Geometry: final body of the model. Coordinates: model frame, mm. Face numbers are marked on the shaded views. A direction names the side the tool comes from. Round coordinates to 2 decimals unless told otherwise and drop trailing zeros. Write each loop counter-clockwise with the first axis right and the second up, starting at its lowest first coordinate (ties: lowest second). Pieces come first, ordered by that corner, then holes. Notation, with made-up numbers: M 10.25,-19 L 40.25,-19 A14 cw 40.25,-6 Z; hole C -6.75,34 d4. An arc over 180 degrees is marked long. Put each result on its own line as item: value. Start each with the question number.
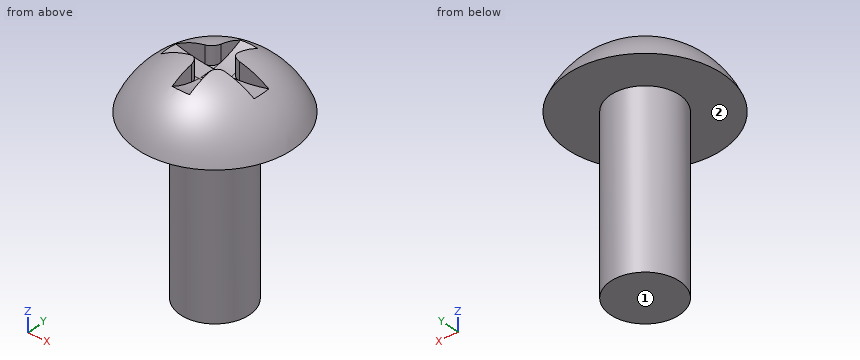
```python
from build123d import *

# Parameters (mm, degrees)
F0_R         = 2
F1_DEPTH     = 10
F5_DEPTH     = 0.5
F7_DEPTH     = 0.5
F8_T4_DEPTH  = 3.6233825309
F8_S5_R      = 10
F8_T6_DEPTH  = 3
F8_S7_R      = 5
F8_T8_DEPTH  = 3
F8_T12_DEPTH = 3.6233825309
F8_S13_R     = 10
F8_T14_DEPTH = 3
F8_S15_R     = 5
F8_T16_DEPTH = 3
F8_T20_DEPTH = 3.6233825309
F8_S21_R     = 10
F8_T22_DEPTH = 3
F8_S23_R     = 5
F8_T24_DEPTH = 3
F8_T28_DEPTH = 3.6233825309
F8_S29_R     = 10
F8_T30_DEPTH = 3
F8_S31_R     = 5
F8_T32_DEPTH = 3


# Not quite as in the source:
# - a fillet or chamfer that OpenCascade refuses, or shapes differently, is made with other operations: its cross-section is extruded or revolved along the edge and cut away or added


with BuildPart() as f1:
    # F0 (on Top) → F1 (new body)
    with BuildSketch(Plane.XY):
        Circle(F0_R)
    extrude(amount=F1_DEPTH)

    # F2 (on Front) → F3 (revolve)
    with BuildSketch(Plane.XZ):
        with BuildLine():
            Line((0, 10), (4.5, 10))
            ThreePointArc((4.5, 10), (2.7041634566, 12.1812451849), (0, 13))
            Line((0, 13), (0, 10))
        make_face()
    revolve(axis=Axis((0, 0, 12.25), (0, 0, -1)))

    # F4 (on Front) → F5 (cut, symmetric)
    with BuildSketch(Plane.XZ):
        with BuildLine():
            ThreePointArc((-2.7226391671, 12.177773856), (0, 11.8), (2.7226391671, 12.177773856))
            ThreePointArc((2.7226391671, 12.177773856), (0, 13), (-2.7226391671, 12.177773856))
        make_face()
    extrude(amount=F5_DEPTH, both=True, mode=Mode.SUBTRACT)

    # F6 (on Right) → F7 (cut, symmetric)
    with BuildSketch(Plane.YZ):
        with BuildLine():
            ThreePointArc((-2.3644931313, 12.3944157899), (0, 11.8), (2.3644931313, 12.3944157899))
            ThreePointArc((2.3644931313, 12.3944157899), (0, 13), (-2.3644931313, 12.3944157899))
        make_face()
    extrude(amount=F7_DEPTH, both=True, mode=Mode.SUBTRACT)

    # F8: fillet of radius 0.5 on 4 edges, made by hand


with BuildPart() as f8_tool2:
    # F8_s3 → F8_t4 (new body)
    with BuildSketch(Plane.XY.offset(10.5750628145)):
        with BuildLine():
            ThreePointArc((1, -0.5), (0.6464466094, -0.6464466094), (0.5, -1))
            Line((0.5, -1), (0.5, -0.5))
            Line((0.5, -0.5), (1, -0.5))
        make_face()
    extrude(amount=F8_T4_DEPTH)

    # F8_s5 → F8_t6 (intersect, symmetric)
    with BuildSketch(Plane.XZ.offset(0.8)):
        with Locations((0, 21.8)):
            Circle(F8_S5_R)
    extrude(amount=F8_T6_DEPTH, both=True, mode=Mode.INTERSECT)

    # F8_s7 → F8_t8 (intersect, symmetric)
    with BuildSketch(Plane.YZ.offset(0.8)):
        with Locations((0, 16.8)):
            Circle(F8_S7_R)
    extrude(amount=F8_T8_DEPTH, both=True, mode=Mode.INTERSECT)


with BuildPart() as f1_1:
    add(f1.part)

    # F8_t1: cut F8_tool2
    add(f8_tool2.part, mode=Mode.SUBTRACT)


with BuildPart() as f8_tool10:
    # F8_s11 → F8_t12 (new body)
    with BuildSketch(Plane.XY.offset(10.5750628145)):
        with BuildLine():
            ThreePointArc((-1, -0.5), (-0.6464466094, -0.6464466094), (-0.5, -1))
            Line((-0.5, -1), (-0.5, -0.5))
            Line((-0.5, -0.5), (-1, -0.5))
        make_face()
    extrude(amount=F8_T12_DEPTH)

    # F8_s13 → F8_t14 (intersect, symmetric)
    with BuildSketch(Plane.XZ.offset(0.8)):
        with Locations((0, 21.8)):
            Circle(F8_S13_R)
    extrude(amount=F8_T14_DEPTH, both=True, mode=Mode.INTERSECT)

    # F8_s15 → F8_t16 (intersect, symmetric)
    with BuildSketch(Plane.YZ.offset(-0.8)):
        with Locations((0, 16.8)):
            Circle(F8_S15_R)
    extrude(amount=F8_T16_DEPTH, both=True, mode=Mode.INTERSECT)


with BuildPart() as f1_2:
    add(f1_1.part)

    # F8_t9: cut F8_tool10
    add(f8_tool10.part, mode=Mode.SUBTRACT)


with BuildPart() as f8_tool18:
    # F8_s19 → F8_t20 (new body)
    with BuildSketch(Plane.XY.offset(10.5750628145)):
        with BuildLine():
            ThreePointArc((-1, 0.5), (-0.6464466094, 0.6464466094), (-0.5, 1))
            Line((-0.5, 1), (-0.5, 0.5))
            Line((-0.5, 0.5), (-1, 0.5))
        make_face()
    extrude(amount=F8_T20_DEPTH)

    # F8_s21 → F8_t22 (intersect, symmetric)
    with BuildSketch(Plane.XZ.offset(-0.7)):
        with Locations((0, 21.8)):
            Circle(F8_S21_R)
    extrude(amount=F8_T22_DEPTH, both=True, mode=Mode.INTERSECT)

    # F8_s23 → F8_t24 (intersect, symmetric)
    with BuildSketch(Plane.YZ.offset(-0.8)):
        with Locations((0, 16.8)):
            Circle(F8_S23_R)
    extrude(amount=F8_T24_DEPTH, both=True, mode=Mode.INTERSECT)


with BuildPart() as f1_3:
    add(f1_2.part)

    # F8_t17: cut F8_tool18
    add(f8_tool18.part, mode=Mode.SUBTRACT)


with BuildPart() as f8_tool26:
    # F8_s27 → F8_t28 (new body)
    with BuildSketch(Plane.XY.offset(10.5750628145)):
        with BuildLine():
            ThreePointArc((1, 0.5), (0.6464466094, 0.6464466094), (0.5, 1))
            Line((0.5, 1), (0.5, 0.5))
            Line((0.5, 0.5), (1, 0.5))
        make_face()
    extrude(amount=F8_T28_DEPTH)

    # F8_s29 → F8_t30 (intersect, symmetric)
    with BuildSketch(Plane.XZ.offset(-0.7)):
        with Locations((0, 21.8)):
            Circle(F8_S29_R)
    extrude(amount=F8_T30_DEPTH, both=True, mode=Mode.INTERSECT)

    # F8_s31 → F8_t32 (intersect, symmetric)
    with BuildSketch(Plane.YZ.offset(0.8)):
        with Locations((0, 16.8)):
            Circle(F8_S31_R)
    extrude(amount=F8_T32_DEPTH, both=True, mode=Mode.INTERSECT)


with BuildPart() as f1_4:
    add(f1_3.part)

    # F8_t25: cut F8_tool26
    add(f8_tool26.part, mode=Mode.SUBTRACT)


solid = f1_4.part
```
1) Section A-A, the plane y = -0.75. Output: boundary loops of the cut face in (x, z) (3 decimals).
2) Section D-D, the plane y = -1.75. Output: boundary loops of the cut face in (x, z) (3 decimals).
3) First-contact query: pin 1 (0.5 mm diameter, centred on y = -1.5, z = 12.5, fed in from +X); pin 2 (1.5 mm diameter, centred on x = 3, y = -1.5, fed in from -Z); pin 3 (3 mm diameter, centred on y = 1.5, z = 7.5, fed in from +X). Flat tips, straight axial feed; report the tip coordinate or a pass-through.
4) Section B-B, the plane x = 2.25. Output: boundary loops of the cut face in (y, z) (3 decimals), and give its area (3 significant figures).
5) Ray query, probe 1 along Z at (x, y) = (1, -2.5); probe 2 along Z at (x, y) = (1.25, 2); probe 3 along X at (y, z) = (-2.5, 10.75). Return the intervals inside material, ascending.
6) Section C-C, the plane z = 7.75. Output: boundary loops of the cut face in (x, y), and give its area (3 significant figures).
7) Access query for the marked faces 1 and 2. Directions: +Z, -Z, +X, -X, +Y, -Y. A direction counts if a zero-diameter tool reaches every point of the face in a straight line with its end or side. Return the directions, or none.
Solved:
1. outline: M -4.437,10 L -1.854,10 L -1.854,0 L 1.854,0 L 1.854,10 L 4.437,10 A4.817 ccw 0.567,12.908 L 0.567,11.857 L -0.567,11.857 L -0.567,12.908 A4.817 ccw Z
2. outline: M -4.146,10 L -0.968,10 L -0.968,0 L 0.968,0 L 0.968,10 L 4.146,10 A4.55 ccw 0.5,12.648 L 0.5,12.116 L -0.5,12.116 L -0.5,12.648 A4.55 ccw Z
3. pin 1: stops at x = 2.15
3. pin 2: stops at z = 10
3. pin 3: stops at x = 2
4. outline: M -3.897,10 L 3.897,10 A4.325 ccw 0.5,12.421 L 0.5,12.056 L -0.5,12.056 L -0.5,12.421 A4.325 ccw Z
4. area: 13.3 mm2
5. probe 1: z = 10 to 12.19
5. probe 2: z = 10 to 12.39
5. probe 3: x = -3.26 to 3.26
6. outline: C 0,0 d4
6. area: 12.6 mm2
7. face 1: -Z, +X, -X, +Y, -Y
7. face 2: -Z
